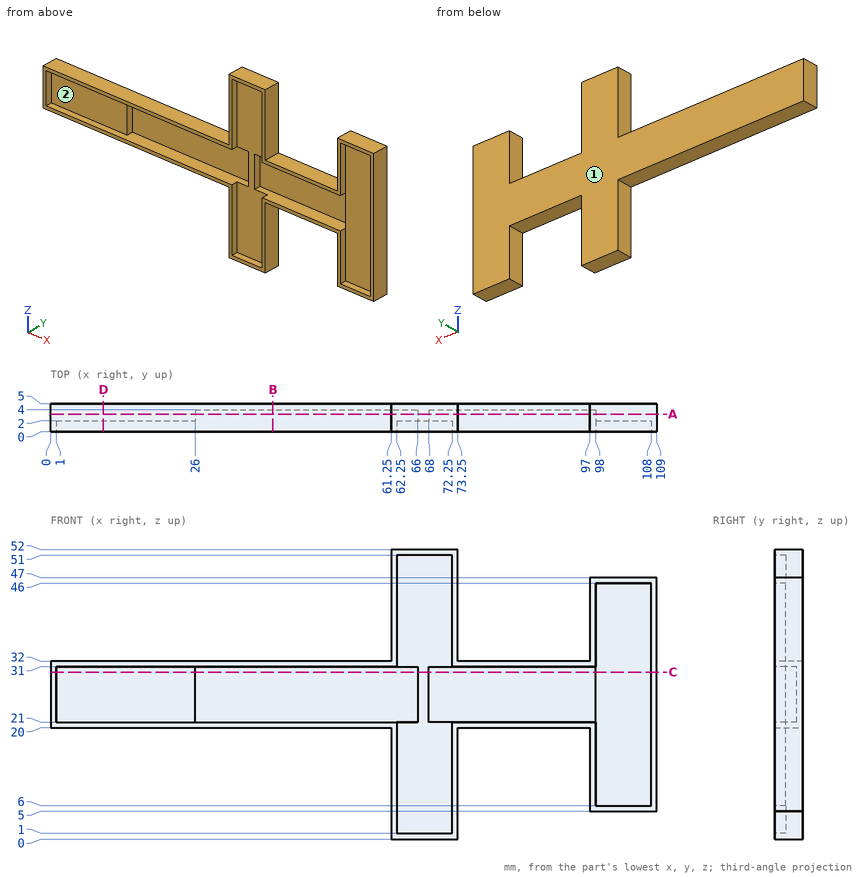
Input: dimensioned drawing with shaded views. Units: mm. Origin: part minimum x, y, z. Round coordinates to 2 decimals unless told otherwise and drop trailing zeros. Write each loop counter-clockwise with the first axis right and the second up, starting at its lowest first coordinate (ties: lowest second). Pieces come first, ordered by that corner, then holes. Notation, with made-up numbers: (-36.75, 13.5) -> (-16.75, 13.5) arc R20 ccw to (-16.75, 39.5) -> close; hole circle Ø9 at (-31.5, 39). An arc over 180 degrees is marked (long way). Use CSV: the item, a comma, the result in double quotes. Start each with the question number.
Q1. First-contact query: pin 1 Ø0.6 at (y, z) = (1, 42) entering from -X; pin 2 Ø1.2 at (x, y) = (89, 1.5) entering from -Z; pin 3 Ø2.5 at (x, y) = (84, 2) entering from +Z. Flat tips, straight axial feed; report the tip coordinate or a pass-through.
Q2. Pull-direction query (Z, two-part tool) for the marked faces 1 and 2; classes: pulls with the +Z half, pulls with the -Z half, needs draft (parallel to the pull), parting line crosses it, or undercut.
Q3. Section D-D (x = 9.5). Return loops of the section in (y, z), plus the area to 3 significant figures.
Q4. Section A-A (y = 3.2). Return loops of the section in (x, z), plus the area to 3 significant figures.
Q5. Section B-B (x = 40). Return loops of the section in (y, z).
Q6. Section C-C (z = 30). Return loops of the section in (x, y), plus the area to 3 significant figures.
Q7. Line query: L1, parallel to X at y = 3.2, z = 27; L2, parallel to X at y = 1.65, z = 11; L3, parallel to X at y = 0.75, z = 4. Output: solid intervals per line, ascending.
Result sheet:
1,pin 1,"x = 61.25"
1,pin 2,"z = 20"
1,pin 3,"z = 32"
2,face 1,"needs draft"
2,face 2,"undercut"
3,outline,"(0, 20) -> (5, 20) -> (5, 32) -> (0, 32) -> (0, 31) -> (2, 31) -> (2, 21) -> (0, 21) -> close"
3,area,"40.0 mm²"
4,outline,"(0, 20) -> (61.25, 20) -> (61.25, 0) -> (73.25, 0) -> (73.25, 20) -> (97, 20) -> (97, 5) -> (109, 5) -> (109, 47) -> (97, 47) -> (97, 32) -> (73.25, 32) -> (73.25, 52) -> (61.25, 52) -> (61.25, 32) -> (0, 32) -> close; hole (26, 21) -> (66, 21) -> (66, 31) -> (26, 31) -> close; hole (68, 21) -> (98, 21) -> (98, 31) -> (68, 31) -> close"
4,area,"1,450 mm²"
5,outline,"(0, 20) -> (5, 20) -> (5, 32) -> (0, 32) -> (0, 31) -> (4, 31) -> (4, 21) -> (0, 21) -> close"
6,outline,"(0, 0) -> (1, 0) -> (1, 2) -> (26, 2) -> (26, 4) -> (66, 4) -> (66, 2) -> (68, 2) -> (68, 4) -> (98, 4) -> (98, 2) -> (108, 2) -> (108, 0) -> (109, 0) -> (109, 5) -> (0, 5) -> close"
6,area,"191 mm²"
7,L1,"0 to 26, 66 to 68, 98 to 109"
7,L2,"61.25 to 62.25, 72.25 to 73.25, 97 to 98, 108 to 109"
7,L3,"61.25 to 62.25, 72.25 to 73.25"
